Source: CAD feature listing. Evaluate the final solid. Frame: model axes, mm. Face numbers are marked on the shaded views. A direction names the side the tool comes from. Give positions to 0.01 mm unless a question says otherwise; leave off trailing zeros. Loops run counter-clockwise (first coordinate to the right, second up) from the corner with the lowest first, then second, coordinate; pieces in that order, holes last. Notation, with made-up numbers: M 74.25,-0.5 L 115.25,-0.5 A35 cw 115.25,37.5 Z; hole C 73,-36.5 d3. An arc over 180 degrees is marked long. Write item = value, one per line.
from build123d import *

# Parameters (mm, degrees)
PAD008_DEPTH       = 40
SKETCH033_W        = 30
SKETCH033_H        = 13.5
POCKET020_DEPTH    = 21.001
POCKET021_DEPTH    = 37.501
SKETCH035_R        = 8
POCKET022_DEPTH    = 13.001
SKETCH036_R        = 3.15
POCKET023_DEPTH    = 8.001
SKETCH037_W        = 11
SKETCH037_H        = 24
POCKET024_DEPTH    = 8.001
FILLET003002004_R  = 8
SKETCH038_R        = 2
POCKET025_DEPTH    = 37.501
SKETCH039_R        = 2.55
POCKET026_DEPTH    = 6
SKETCH040_W        = 10
SKETCH040_H        = 8
POCKET027_DEPTH    = 1
CHAMFER026013_SIZE = 2
CHAMFER026014_SIZE = 0.4
CHAMFER026015_SIZE = 0.99
CHAMFER026016_SIZE = 0.5


with BuildPart() as part:
    # Sketch032 → Pad008 (new body)
    with BuildSketch(Plane.XZ):
        Polygon((-20, 10.5), (-10, 10.5), (-10, 2), (0, -3), (0, -11.1), (1, -11.1), (1, -18.9), (0, -18.9), (0, -27), (-20, -27), align=None)
    extrude(amount=PAD008_DEPTH)

    # Sketch033 (on DatumPlane) → Pocket020 (cut, through all)
    with BuildSketch(Plane.YZ.offset(-20)):
        with Locations((-15, 3.75)):
            Rectangle(SKETCH033_W, SKETCH033_H)
    extrude(amount=POCKET020_DEPTH, mode=Mode.SUBTRACT)

    # Sketch034 (on DatumPlane) → Pocket021 (cut, through all)
    with BuildSketch(Plane.XY.offset(-27)):
        Polygon((-20, -30), (-7, -25), (-7, 0), (-20, 0), align=None)
    extrude(amount=POCKET021_DEPTH, mode=Mode.SUBTRACT)

    # Sketch035 (on DatumPlane) → Pocket022 (cut, through all)
    with BuildSketch(Plane.YZ.offset(-7)):
        with Locations((-21, -15)):
            Circle(SKETCH035_R)
    extrude(amount=-POCKET022_DEPTH, mode=Mode.SUBTRACT)

    # Sketch036 (on DatumPlane) → Pocket023 (cut, through all)
    with BuildSketch(Plane.YZ.offset(-7)):
        with Locations((-21, -15)):
            Circle(SKETCH036_R)
    extrude(amount=POCKET023_DEPTH, mode=Mode.SUBTRACT)

    # Sketch037 (on DatumPlane) → Pocket024 (cut, through all)
    with BuildSketch(Plane.YZ.offset(-7)):
        with Locations((-5.5, -15)):
            Rectangle(SKETCH037_W, SKETCH037_H)
    extrude(amount=POCKET024_DEPTH, mode=Mode.SUBTRACT)

    # Fillet003002004
    fillet003002004_edges = [part.edges().sort_by_distance(p)[0] for p in [
        (-3.5, -11, -27),
        (-3.5, -11, -3),
    ]]
    fillet(fillet003002004_edges, radius=FILLET003002004_R)

    # Sketch038 (on DatumPlane) → Pocket025 (cut, through all)
    with BuildSketch(Plane.XY.offset(10.5)):
        with Locations((-15, -35)):
            Circle(SKETCH038_R)
    extrude(amount=-POCKET025_DEPTH, mode=Mode.SUBTRACT)

    # Sketch039 (on DatumPlane) → Pocket026 (cut)
    with BuildSketch(Plane.XY.offset(10.5)):
        with Locations((-15, -35)):
            Circle(SKETCH039_R)
    extrude(amount=-POCKET026_DEPTH, mode=Mode.SUBTRACT)

    # Sketch040 (on DatumPlane) → Pocket027 (cut)
    with BuildSketch(Plane.YZ.offset(1)):
        with Locations((-21, -15)):
            Rectangle(SKETCH040_W, SKETCH040_H)
    extrude(amount=-POCKET027_DEPTH, mode=Mode.SUBTRACT)

    # Chamfer026013
    chamfer026013_edges = [part.edges().sort_by_distance(p)[0] for p in [
        (-10, -40, 6.25),
        (-20, -40, -8.25),
        (-10, -30, 6.25),
        (-20, -30, 3.75),
    ]]
    chamfer(chamfer026013_edges, length=CHAMFER026013_SIZE)

    # Chamfer026014
    chamfer026014_edges = [part.edges().sort_by_distance(p)[0] for p in [
        (-9, -40, -27),
        (0, -40, -22.95),
        (0.5, -40, -18.9),
        (1, -40, -15),
        (0.5, -40, -11.1),
        (0, -40, -7.05),
        (-19, -39, -27),
        (-20, -34, -27),
        (-13.5, -27.5, -27),
        (-7, -22, -27),
        (-7, -13.343146, -24.656854),
        (-7, -11, -15),
        (-7, -13.343146, -5.343146),
        (-7, -22, -3),
        (-13.5, -27.5, -3),
        (-20, -31, -3),
        (-7, -24.15, -15),
        (0, -24.15, -15),
        (-17, -35, -27),
        (-15, -40, 10.5),
        (-19, -39, 10.5),
        (-20, -35, 10.5),
        (-19, -31, 10.5),
        (-15, -30, 10.5),
        (-11, -31, 10.5),
        (-10, -35, 10.5),
        (-11, -39, 10.5),
        (-17.55, -35, 10.5),
        (-5, -40, -0.5),
        (-11, -40, 2.5),
    ]]
    chamfer(chamfer026014_edges, length=CHAMFER026014_SIZE)

    # Chamfer026015
    chamfer026015_edges = [part.edges().sort_by_distance(p)[0] for p in [
        (1, -16, -15),
    ]]
    chamfer(chamfer026015_edges, length=CHAMFER026015_SIZE)

    # Chamfer026016
    chamfer026016_edges = [part.edges().sort_by_distance(p)[0] for p in [
        (-17, -35, 4.5),
    ]]
    chamfer(chamfer026016_edges, length=CHAMFER026016_SIZE)


with BuildPart() as part_1:
    # Body001001001002003006 placement: moved
    add(part.part.moved(Location((10, -25, 0))))


solid = part_1.part
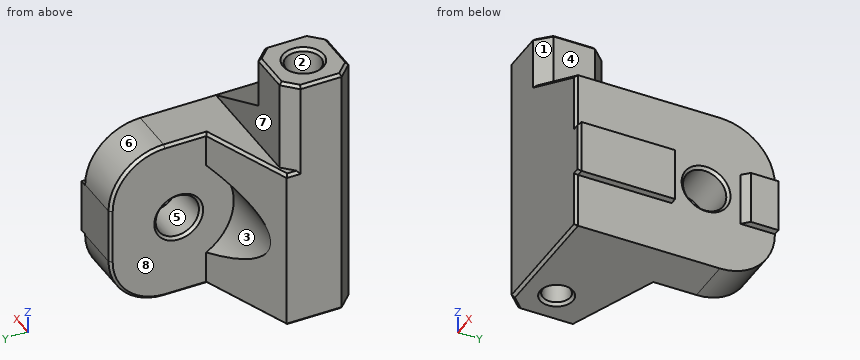
1. Pull-direction query (Z, two-part tool) for the marked faces 5, 6, 7 and 8; classes: +Z half, -Z half, draft (parallel to the pull), parting line (faces both ways), or undercut.
Derived:
face_5 = undercut
face_6 = +Z half
face_7 = draft
face_8 = undercut
2. Cut plane A-A, the plane y = -60. Return the cut outline in (x, z).
Derived:
outline = M -10,-26.6 L -9.6,-27 L -7.4,-27 L -7,-26.6 L -7,4 L -7.5,4.5 L -7.55,4.5 L -7.55,10.1 L -7.95,10.5 L -9.6,10.5 L -10,10.1 Z; M -3,-26.6 L -2.6,-27 L 10,-27 L 10,-18.9 L 11,-18.9 L 11,-11.1 L 10,-11.1 L 10,-3 L 0,2 L 0,10.1 L -0.4,10.5 L -2.05,10.5 L -2.45,10.1 L -2.45,4.5 L -2.5,4.5 L -3,4 Z
3. First-contact query: pin 1 Ø0.8 at (x, y) = (10.5, -57) entering from -Z; pin 2 Ø8 at (x, z) = (-2, -9) entering from +Y; pin 3 Ø7 at (y, z) = (-47, -17.5) entering from +X; pin 4 Ø12 at (y, z) = (-53, -7) entering from +X. Flat tips, straight axial feed; report the tip coordinate or a pass-through.
Derived:
pin_1 = -18.9
pin_2 = -50.41
pin_3 = 10
pin_4 = 11
4. Cut plane C-C, the plane x = -5. Return the cut outline in (y, z), then the cut area to 3 significant figures.
Derived:
outline = M -65,-26.6 L -64.6,-27 L -62.4,-27 L -62,-26.6 L -62,4 L -62.5,4.5 L -62.55,4.5 L -62.55,10.1 L -62.95,10.5 L -64.6,10.5 L -65,10.1 Z; M -58,-26.6 L -57.6,-27 L -53.51,-27 L -53.08,-26.6 L -53.08,-18.73 A8 cw -53.08,-11.27 L -53.08,-3.4 L -53.51,-3 L -55,-3 L -55,10.1 L -55.4,10.5 L -57.05,10.5 L -57.45,10.1 L -57.45,4.5 L -57.5,4.5 L -58,4 Z
area = 259 mm²
5. Cut plane D-D, the plane y = -46. Return the cut outline in (x, z), then the cut area to 3 significant figures.
Derived:
outline = M 3,-26.6 L 3.4,-27 L 10,-27 L 10,-18.55 L 9.6,-18.15 L 3.4,-18.15 L 3,-18.55 Z; M 3,-11.45 L 3.4,-11.85 L 9.6,-11.85 L 10,-11.45 L 10,-3 L 3.4,-3 L 3,-3.4 Z
area = 123 mm²
6. Material intervals for probe 1 along Y at (x, z) = (4.75, -15); probe 2 along Z at (x, y) = (5.75, -46); probe 3 along X at (y, z) = (-52.5, -13.5), sorted ascending. Write a range as from..to.
Derived:
probe_1 = -65..-49.15, -42.85..-36
probe_2 = -27..-18.15, -11.85..-3
probe_3 = 3..11
7. Reachability of the marked faces 1, 2, 3 and 4 from +Z, -Z, +X, -X, +Y, -Y: full face, straight path, thin tool, end or side. Return the list, or none.
Derived:
face_1 = +Z, +X, -Y
face_2 = +Z
face_3 = -X, +Y
face_4 = +Z, +X, +Y, -Y
8. Cut plane B-B, the plane z = -15. Count the separate pieces of the cut face and the enclosed holes in it, then the cut area to 3 significant figures.
Derived:
separate_pieces = 2
enclosed_holes = 1
area = 304 mm²
